```python
from build123d import *

# Parameters (mm, degrees)
BOSS_EXTRUDE1_DEPTH = 3


with BuildPart() as part:
    # Sketch1 → Boss-Extrude1 (new body)
    with BuildSketch(Plane(origin=(0, 0, 0), x_dir=(0, 0, -1), z_dir=(1, 0, 0))):
        with BuildLine():
            Line((-32.5, 50), (-32.5, 0))
            Line((-32.5, 0), (-15, 0))
            ThreePointArc((-15, 0), (0, 15), (15, 0))
            Line((15, 0), (32.5, 0))
            Line((32.5, 0), (32.5, 50))
            Line((32.5, 50), (10.84, 50))
            Line((10.84, 50), (10.84, 47))
            Line((10.84, 47), (-10.84, 47))
            Line((-10.84, 47), (-10.84, 50))
            Line((-10.84, 50), (-32.5, 50))
        make_face()
    extrude(amount=BOSS_EXTRUDE1_DEPTH)


solid = part.part
```
Source: CAD feature listing. Evaluate the final solid. Frame: model axes, mm. A direction names the side the tool comes from. Give positions to 0.01 mm unless a question says otherwise; leave off trailing zeros. Loops run counter-clockwise (first coordinate to the right, second up) from the corner with the lowest first, then second, coordinate; pieces in that order, holes last. Notation, with made-up numbers: (16, 35) -> (53, 35) arc R21 ccw to (53, 42) -> close; hole circle Ø10 at (57, 14). An arc over 180 degrees is marked (long way). Use a Markdown table: item, result. Add a question column.
(1) Section query B-B (y = 7). Output: boundary loops of the cut face in (x, z).
(2) Section query A-A (x = 0.6). Output: boundary loops of the cut face in (y, z).
(3) Section query D-D (z = 13). Output: boundary loops of the cut face in (x, y).
(4) Access query for faces 1 (the face through (1, 0, 24)), 2 (the face through (1, 47, 0)). Directions: +Z, -Z, +X, -X, +Y, -Y. A direction counts if a zero-diameter tool reaches every point of the face in a straight line with its end or side. Return the directions, or none.
(5) Ray query, line 1 (Z direction, x = 1.75, y = 13); line 2 (Z direction, x = 1.25, y = 7.5); line 3 (Y direction, x = 1.5, z = -2). Return the intervals inside material, ascending.
(6) Pull-direction query (Z, two-part tool) for faces 3 (the face through (1, 25, -32.5)), 4 (the face through (1, 48, 10.84)), 5 (the face through (0, 25, 0)), 6 (the face through (1, 25, 32.5)); classes: +Z half, -Z half, draft (parallel to the pull), parting line (faces both ways), or undercut.
(7) Section query C-C (z = 0). Output: boundary loops of the cut face in (x, y), then the cut area to 3 significant figures.
Checked values:
| question | item | result |
|---|---|---|
| 1 | outline | (0, -32.5) -> (3, -32.5) -> (3, -13.27) -> (0, -13.27) -> close; (0, 13.27) -> (3, 13.27) -> (3, 32.5) -> (0, 32.5) -> close |
| 2 | outline | (0, -32.5) -> (50, -32.5) -> (50, -10.84) -> (47, -10.84) -> (47, 10.84) -> (50, 10.84) -> (50, 32.5) -> (0, 32.5) -> (0, 15) arc R15 cw to (0, -15) -> close |
| 3 | outline | (0, 7.48) -> (3, 7.48) -> (3, 50) -> (0, 50) -> close |
| 4 | face 1 | +Z, -Z, +X, -X, -Y |
| 4 | face 2 | +X, -X, +Y |
| 5 | line 1 | -32.5 to -7.48, 7.48 to 32.5 |
| 5 | line 2 | -32.5 to -12.99, 12.99 to 32.5 |
| 5 | line 3 | 14.87 to 47 |
| 6 | face 3 | -Z half |
| 6 | face 4 | undercut |
| 6 | face 5 | draft |
| 6 | face 6 | +Z half |
| 7 | outline | (0, 15) -> (3, 15) -> (3, 47) -> (0, 47) -> close |
| 7 | area | 96.0 mm^2 |
